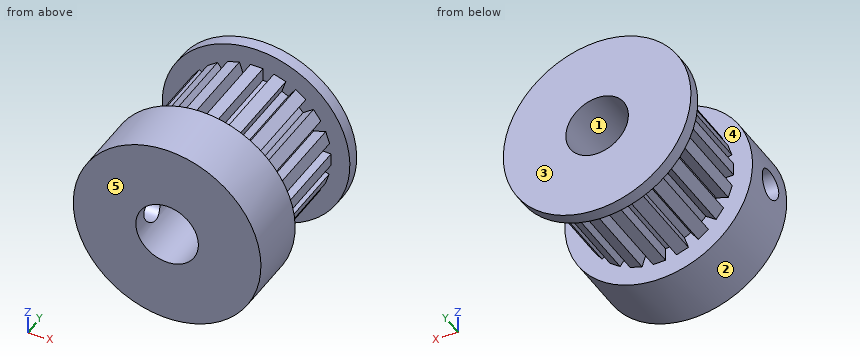
```python
from build123d import *

# Parameters (mm, degrees)
IZIM1_R                     = 7.5
Y_KSEKLIK_EKSTR_ZYON1_DEPTH = 5
IZIM6_R                     = 5
Y_KSEKLIK_EKSTR_ZYON5_DEPTH = 8
Y_KSEKLIK_EKSTR_ZYON6_START = -8
Y_KSEKLIK_EKSTR_ZYON6_DEPTH = 8
DAIRESEL_KAPLAMA2_COUNT     = 20
IZIM8_R                     = 7.5
Y_KSEKLIK_EKSTR_ZYON7_DEPTH = 1
IZIM9_R                     = 2.5
KES_EKSTR_ZYON2_DEPTH       = 21
IZIM10_R                    = 1.2
KES_EKSTR_ZYON3_DEPTH       = 21


with BuildPart() as part:
    # Çizim1 → Yükseklik-Ekstrüzyon1 (new body)
    with BuildSketch(Plane(origin=(0, 0, 0), x_dir=(1, 0, 0), z_dir=(0, 1, 0))):
        with Locations(Location((0, 0, 0), (0, 0, 270))):
            Circle(IZIM1_R)
    extrude(amount=Y_KSEKLIK_EKSTR_ZYON1_DEPTH)

    # Çizim6 → Yükseklik-Ekstrüzyon5 (add)
    with BuildSketch(Plane(origin=(0, 5, 0), x_dir=(1, 0, 0), z_dir=(0, 1, 0))):
        with Locations(Location((0, 0, 0), (0, 0, 270))):
            Circle(IZIM6_R)
    extrude(amount=Y_KSEKLIK_EKSTR_ZYON5_DEPTH)

    # Çizim7 → Yükseklik-Ekstrüzyon6 (add)
    with BuildSketch(Plane(origin=(0, 13, 0), x_dir=(1, 0, 0), z_dir=(0, 1, 0)).offset(Y_KSEKLIK_EKSTR_ZYON6_START)):
        with BuildLine():
            Line((0, 6), (0, 5))
            ThreePointArc((0, 5), (0.223628846, 4.99499651), (0.446810123, 4.979996056))
            Line((0.446810123, 4.979996056), (0.446810123, 6))
            Line((0.446810123, 6), (0, 6))
        make_face()
        with BuildLine():
            ThreePointArc((-0.553189877, 4.969303871), (-0.277020438, 4.99232007), (0, 5))
            Line((0, 5), (0, 6))
            Line((0, 6), (-0.553189877, 6))
            Line((-0.553189877, 6), (-0.553189877, 4.969303871))
        make_face()
    y_kseklik_ekstr_zyon6 = extrude(amount=Y_KSEKLIK_EKSTR_ZYON6_DEPTH)

    # Dairesel Kaplama2: Yükseklik-Ekstrüzyon6 ×20 about axis
    dairesel_kaplama2_axis = Axis((0, 0, 0), (0, 1, 0))
    for i in range(1, DAIRESEL_KAPLAMA2_COUNT):
        add(y_kseklik_ekstr_zyon6.rotate(dairesel_kaplama2_axis, i * 360 / DAIRESEL_KAPLAMA2_COUNT))

    # Çizim8 → Yükseklik-Ekstrüzyon7 (add)
    with BuildSketch(Plane(origin=(0, 13, 0), x_dir=(1, 0, 0), z_dir=(0, 1, 0))):
        with Locations(Location((0, 0, 0), (0, 0, 270))):
            Circle(IZIM8_R)
    extrude(amount=Y_KSEKLIK_EKSTR_ZYON7_DEPTH)

    # Çizim9 → Kes-Ekstrüzyon2 (cut)
    with BuildSketch(Plane(origin=(0, 14, 0), x_dir=(1, 0, 0), z_dir=(0, 1, 0))):
        with Locations(Location((0, 0, 0), (0, 0, 270))):
            Circle(IZIM9_R)
    extrude(amount=-KES_EKSTR_ZYON2_DEPTH, mode=Mode.SUBTRACT)

    # Çizim10 → Kes-Ekstrüzyon3 (cut)
    with BuildSketch(Plane(origin=(0, 0, 0), x_dir=(0, 0, -1), z_dir=(1, 0, 0))):
        with Locations((0, 2.361227205)):
            Circle(IZIM10_R)
    extrude(amount=-KES_EKSTR_ZYON3_DEPTH, mode=Mode.SUBTRACT)


solid = part.part
```
Can you work these out from the model? Positions are in its coordinate system, mm. Face numbers are marked on the shaded views. A direction names the side the tool comes from. Give positions to 0.01 mm unless a question says otherwise; leave off trailing zeros. Loops run counter-clockwise (first coordinate to the right, second up) from the corner with the lowest first, then second, coordinate; pieces in that order, holes last. Notation, with made-up numbers: M 45,44 L 49,44 A24 cw 49,83 Z; hole C 66.25,71 d8. An arc over 180 degrees is marked long. Use CSV: the item, a comma, the result in double quotes. Start each with the question number.
1. Imagine slicing it at B-B, the plane x = 0. Write out the boundary of the cut face in (y, z), plus the area to 3 significant figures.
2. For P1, Ø0.8, axis at x = 5.5, y = 10.5, coming from the +Z side; P2, Ø5, axis at y = 4, z = -3.5, coming from the -X side; P3, Ø0.5, axis at x = -0.5, y = 8.5, coming from the -Z side, each with a flat end and sliding along its axis, tell me the tip position at first contact or that it passes through.
3. Imagine slicing it at A-A, the plane z = 0. Write out the boundary of the cut face in (x, y), plus the area to 3 significant figures.
4. On a 3-axis mill with a long thin cutter (end or side, diameter ignored), from which of +Z, -Z, +X, -X, +Y, -Y can I reach the whole of each face in a straight line? I mean the marked faces 4 and 5. Say none if no direction works.
5. Imagine slicing it at C-C, the plane y = 4.5. Write out the boundary of the cut face in (x, z).
6. If we mould it in two halves opening along Z, with no side actions, what happens to the marked faces 1, 2 and 3? For each: released by +Z, released by -Z, zero draft, split by the parting line, or undercut.
7. Imagine slicing it at D-D, the plane x = 6.5. Write out the boundary of the cut face in (y, z), plus the area to 3 significant figures.
8. If I drill on L1, parallel to Y at x = -6.1, z = 0; L2, parallel to Y at x = 3.75, z = -5.25; L3, parallel to Y at x = -5.4, z = 0, over which ranges is the centre line in solid material (lowest first)?
Response values:
1,outline,"M 0,-7.5 L 5,-7.5 L 5,-6 L 13,-6 L 13,-7.5 L 14,-7.5 L 14,-2.5 L 0,-2.5 Z; M 0,2.5 L 14,2.5 L 14,7.5 L 13,7.5 L 13,6 L 5,6 L 5,7.5 L 0,7.5 Z"
1,area,"116 mm^2"
2,P1,"z = 3.19"
2,P2,"x = -7.43"
2,P3,"z = -6"
3,outline,"M -7.5,0 L -2.5,0 L -2.5,1.16 L -7.5,1.16 Z; M -7.5,3.56 L -2.5,3.56 L -2.5,14 L -7.5,14 L -7.5,13 L -6,13 L -6,5 L -7.5,5 Z; M 2.5,0 L 7.5,0 L 7.5,5 L 6,5 L 6,13 L 7.5,13 L 7.5,14 L 2.5,14 Z"
3,area,"104 mm^2"
4,face 4,"none"
4,face 5,"+Z, -Z, +X, -X, -Y"
5,outline,"C 0,0 d15; hole C 0,0 d5"
6,face 1,"undercut"
6,face 2,"split by the parting line"
6,face 3,"zero draft"
7,outline,"M 0,-3.74 L 5,-3.74 L 5,3.74 L 0,3.74 Z; M 13,-3.74 L 14,-3.74 L 14,3.74 L 13,3.74 Z"
7,area,"44.9 mm^2"
8,L1,"0 to 1.16, 3.56 to 5, 13 to 14"
8,L2,"0 to 5, 13 to 14"
8,L3,"0 to 1.16, 3.56 to 14"
